Input: part model. Units: mm. Frame: model coordinates. A direction names the side the tool comes from. Round coordinates to 2 decimals unless told otherwise and drop trailing zeros. Loops run counter-clockwise (first coordinate to the right, second up) from the corner with the lowest first, then second, coordinate; pieces in that order, holes last. Notation, with made-up numbers: (35, 73) -> (61, 73) arc R22 cw to (61, 87) -> close; hole circle Ø5 at (-38, 76.25). An arc over 180 degrees is marked (long way). One line per question, with ' | ' between items. Start each with the question number.
Q1. Contact query for flat-ended pins moving along their axis: P1, Ø4, axis at x = -405, y = 485.5, coming from the -Z side; P2, Ø4, axis at x = 168.5, y = 438.5, coming from the +Z side; P3, Ø2, axis at y = 336, z = -186, coming from the -X side; P4, Ø5, axis at y = 449.5, z = -282, coming from the -X side. Output: stop coordinate, or through.
Q2. Material intervals for L1, parallel to Z at x = 177, y = 430 (3 decimals); L2, parallel to Z at x = 22.5, y = 928; L3, parallel to X at y = 801.5, z = -27.5, sorted ascending.
Q3. Cut plane A-A on y = 282. Return loops of the section in (x, z) (3 decimals), and give its area (3 significant figures).
Q4. Cut plane B-B on y = 456.5. Return loops of the section in (x, z) (3 decimals), and give its area (3 significant figures).
Q5. Mould query, pull axis X, two halves, no side actions, for faces 1 (the face through (-3, 456, 279.4)), 2 (the face through (-3, 204, 250.825)), 3 (the face through (-303.409, 203.53, 123.657)), 4 (the face through (325.6, 456.49, 141.66)). Classes: pulls with the +X half, pulls with the -X half, needs draft (parallel to the pull), parting line crosses it, or undercut.
Q6. Access query for faces 5 (the face through (303.409, 203.53, -123.657)), 6 (the face through (-491.862, 861.466, 228.492)), 7 (the face through (-325.6, 456.49, -141.66)), 8 (the face through (-4, 861, 463.473)), 9 (the face through (3, 200, -254)). Directions: +Z, -Z, +X, -X, +Y, -Y. A direction counts if a zero-diameter tool reaches every point of the face in a straight line with its end or side. Return the directions, or none.
from build123d import *

# Parameters (mm, degrees)
BOSS_EXTRUDE1_DEPTH = 406.4
BOSS_EXTRUDE2_DEPTH = 101.6
BOSS_EXTRUDE3_DEPTH = 304.8
BOSS_EXTRUDE4_DEPTH = 3.175
SHELL3_START        = 3.175
SHELL3_DEPTH        = 1016
SHELL3_START_2      = 714.375
SHELL3_2_DEPTH      = 304.8
SHELL3_START_3      = 409.575
SHELL3_3_DEPTH      = 304.8


with BuildPart() as part:
    # Sketch2 → Boss-Extrude1 (new body)
    with BuildSketch(Plane(origin=(0, 0, 0), x_dir=(1, 0, 0), z_dir=(0, 1, 0))):
        Polygon((-203.2, 254), (-406.4, 0), (-203.2, -254), (203.2, -254), (406.4, 0), (203.2, 254), align=None)
    extrude(amount=BOSS_EXTRUDE1_DEPTH)

    # Sketch3 → Boss-Extrude2 (add)
    with BuildSketch(Plane(origin=(0, 406.4, 0), x_dir=(1, 0, 0), z_dir=(0, 1, 0))):
        Polygon((215.407871126, 279.4), (-215.407871126, 279.4), (-438.927871126, 0), (-215.407871126, -279.4), (215.407871126, -279.4), (438.927871126, 0), align=None)
    extrude(amount=BOSS_EXTRUDE2_DEPTH)

    # Sketch5 → Loft1 section 0
    with BuildSketch(Plane(origin=(0, 711.2, 0), x_dir=(1, 0, 0), z_dir=(0, 1, 0))):
        with BuildLine():
            Line((642.127871126, 0), (291.669837463, 438.072542079))
            Line((291.669837463, 438.072542079), (-291.669837463, 438.072542079))
            Line((-291.669837463, 438.072542079), (-642.127871126, 0))
            Line((-642.127871126, 0), (-291.669837463, -438.072542079))
            Line((-291.669837463, -438.072542079), (291.669837463, -438.072542079))
            Line((291.669837463, -438.072542079), (642.127871126, 0))
        make_face()
    # Sketch4 → Loft1 section 1
    with BuildSketch(Plane(origin=(0, 508, 0), x_dir=(1, 0, 0), z_dir=(0, 1, 0))):
        with BuildLine():
            Line((438.927871126, 0), (215.407871126, 279.4))
            Line((215.407871126, 279.4), (-215.407871126, 279.4))
            Line((-215.407871126, 279.4), (-438.927871126, 0))
            Line((-438.927871126, 0), (-215.407871126, -279.4))
            Line((-215.407871126, -279.4), (215.407871126, -279.4))
            Line((215.407871126, -279.4), (438.927871126, 0))
        make_face()
    loft()

    # Sketch6 → Boss-Extrude3 (add)
    with BuildSketch(Plane(origin=(0, 711.2, 0), x_dir=(1, 0, 0), z_dir=(0, 1, 0))):
        Polygon((303.877708589, -463.472542079), (674.655742252, 0), (303.877708589, 463.472542079), (-303.877708589, 463.472542079), (-674.655742252, 0), (-303.877708589, -463.472542079), align=None)
    extrude(amount=BOSS_EXTRUDE3_DEPTH)

    # Sketch7 → Boss-Extrude4 (add)
    with BuildSketch(Plane(origin=(0, 1016, 0), x_dir=(1, 0, 0), z_dir=(0, 1, 0))):
        Polygon((-340.501321968, -539.672542079), (340.501321968, -539.672542079), (772.239355631, 0), (340.501321968, 539.672542079), (-340.501321968, 539.672542079), (-772.239355631, 0), align=None)
    extrude(amount=BOSS_EXTRUDE4_DEPTH)

    # Shell3: read off the stored shape, not the designer's step
    # Shell3 outline → Shell3 (cut)
    with BuildSketch(Plane(origin=(0, 0, 0), x_dir=(1, 0, 0), z_dir=(0, 1, 0)).offset(SHELL3_START)):
        Polygon((201.674016109, 250.825), (-201.674016109, 250.825), (-402.334016109, 0), (-201.674016109, -250.825), (201.674016109, -250.825), (402.334016109, 0), align=None)
    extrude(amount=SHELL3_DEPTH, mode=Mode.SUBTRACT)

    # Shell3 2 outline → Shell3 2 (cut)
    with BuildSketch(Plane(origin=(0, 0, 0), x_dir=(1, 0, 0), z_dir=(0, 1, 0)).offset(SHELL3_START_2)):
        Polygon((-302.351724698, -460.297542079), (302.351724698, -460.297542079), (670.589758362, 0), (302.351724698, 460.297542079), (-302.351724698, 460.297542079), (-670.589758362, 0), align=None)
        Polygon((-402.334016109, 0), (-201.674016109, 250.825), (201.674016109, 250.825), (402.334016109, 0), (201.674016109, -250.825), (-201.674016109, -250.825), align=None, mode=Mode.SUBTRACT)
    extrude(amount=SHELL3_2_DEPTH, mode=Mode.SUBTRACT)

    # Shell3 3 outline → Shell3 3 (cut)
    with BuildSketch(Plane(origin=(0, 0, 0), x_dir=(1, 0, 0), z_dir=(0, 1, 0)).offset(SHELL3_START_3)):
        Polygon((434.861887235, 0), (213.881887235, 276.225), (-213.881887235, 276.225), (-434.861887235, 0), (-213.881887235, -276.225), (213.881887235, -276.225), align=None)
        Polygon((-402.334016109, 0), (-201.674016109, 250.825), (201.674016109, 250.825), (402.334016109, 0), (201.674016109, -250.825), (-201.674016109, -250.825), align=None, mode=Mode.SUBTRACT)
    extrude(amount=SHELL3_3_DEPTH, mode=Mode.SUBTRACT)

    # Shell3 4: loft between two sections, ruled curve by curve
    shell3_4_from = [
        Edge.make_line((-213.881887235, 509.092780496, -276.225), (-434.861887235, 509.092780496, 0)),
        Edge.make_line((-434.861887235, 509.092780496, 0), (-213.881887235, 509.092780496, 276.225)),
        Edge.make_line((213.881887235, 509.092780496, -276.225), (-213.881887235, 509.092780496, -276.225)),
        Edge.make_line((434.861887235, 509.092780496, 0), (213.881887235, 509.092780496, -276.225)),
        Edge.make_line((213.881887235, 509.092780496, 276.225), (434.861887235, 509.092780496, 0)),
        Edge.make_line((-213.881887235, 509.092780496, 276.225), (213.881887235, 509.092780496, 276.225)),
    ]
    shell3_4_to = [
        Edge.make_line((-290.925320864, 714.375, -436.523482344), (-640.144106739, 714.375, 0)),
        Edge.make_line((-640.144106739, 714.375, 0), (-290.925320864, 714.375, 436.523482344)),
        Edge.make_line((290.925320864, 714.375, -436.523482344), (-290.925320864, 714.375, -436.523482344)),
        Edge.make_line((640.144106739, 714.375, 0), (290.925320864, 714.375, -436.523482344)),
        Edge.make_line((290.925320864, 714.375, 436.523482344), (640.144106739, 714.375, 0)),
        Edge.make_line((-290.925320864, 714.375, 436.523482344), (290.925320864, 714.375, 436.523482344)),
    ]
    shell3_4 = Solid(Shell([*[Face.make_surface_from_curves(shell3_4_from[k], shell3_4_to[k]) for k in range(6)], Face(Wire(shell3_4_from)), Face(Wire(shell3_4_to))]))
    add(shell3_4, mode=Mode.SUBTRACT)


solid = part.part
Results:
1) P1: z = -44.91 | P2: z = 279.4 | P3: x = -258.4 | P4: through
2) L1: -279.4 to -276.225, 276.225 to 279.4 | L2: -463.47 to -460.3, 460.3 to 463.47 | L3: -652.66 to -648.59, 648.59 to 652.66
3) outline: (-406.4, 0) -> (-203.2, -254) -> (203.2, -254) -> (406.4, 0) -> (203.2, 254) -> (-203.2, 254) -> close; hole (-402.334, 0) -> (-201.674, -250.825) -> (201.674, -250.825) -> (402.334, 0) -> (201.674, 250.825) -> (-201.674, 250.825) -> close | area: 6,680 mm^2
4) outline: (-438.928, 0) -> (-215.408, -279.4) -> (215.408, -279.4) -> (438.928, 0) -> (215.408, 279.4) -> (-215.408, 279.4) -> close; hole (-434.862, 0) -> (-213.882, -276.225) -> (213.882, -276.225) -> (434.862, 0) -> (213.882, 276.225) -> (-213.882, 276.225) -> close | area: 7,240 mm^2
5) face 1: needs draft | face 2: undercut | face 3: undercut | face 4: pulls with the +X half
6) face 5: +Y | face 6: +Z, -X, -Y | face 7: -Z, -X, -Y | face 8: +Z, +X, -X, -Y | face 9: -Z, +X, -X, -Y
